Verification items for the finished model (mm, model axes). A direction names the side the tool comes from. Give positions to 0.01 mm unless a question says otherwise; leave off trailing zeros. Order: outer loops, then holes, each group sorted by start corner. A loop starts at its lowest first (then second) coordinate and runs counter-clockwise, first axis right, second up. Notation, with made-up numbers: (83.5, 1.5) - (114.5, 1.5) arc R31 cw to (114.5, 31.5) - close; hole circle Ø11 at (-39, -27). An arc over 180 degrees is marked (long way). Answer as a JSON object with one key per item and string values.
```python
from build123d import *

# Parameters (mm, degrees)
F0_R     = 28.25
F0_R_2   = 27.05
F1_DEPTH = 8
F0_R_3   = 32.25
F0_R_4   = 4.8
F0_R_5   = 4
F2_DEPTH = 0.7
F3_DEPTH = 30
F4_R     = 0.6


with BuildPart() as f1:
    # F0 (on Top) → F1 (new body)
    with BuildSketch(Plane.XY):
        Circle(F0_R)
        Circle(F0_R_2, mode=Mode.SUBTRACT)
    extrude(amount=F1_DEPTH)

    # F0 (on Top) → F2 (join)
    with BuildSketch(Plane.XY):
        Circle(F0_R_3)
        Circle(F0_R, mode=Mode.SUBTRACT)
        Circle(F0_R)
        Circle(F0_R_2, mode=Mode.SUBTRACT)
        Circle(F0_R_2)
        Circle(F0_R_4, mode=Mode.SUBTRACT)
        Circle(F0_R_4)
        Circle(F0_R_5, mode=Mode.SUBTRACT)
    extrude(amount=-F2_DEPTH)

    # F0 (on Top) → F3 (join)
    with BuildSketch(Plane.XY):
        Circle(F0_R_4)
        Circle(F0_R_5, mode=Mode.SUBTRACT)
    extrude(amount=F3_DEPTH)

    # F4
    f4_edges = [f1.edges().sort_by_distance(p)[0] for p in [
        (-28.25, 0, 0),
        (-27.05, 0, 0),
        (-4.8, 0, 0),
    ]]
    fillet(f4_edges, radius=F4_R)


solid = f1.part
```
(1) Section check C-C (z = 2). Record the cut outline in (x, y).
Computed values:
{"outline": "circle Ø56.5 at (0, 0); circle Ø9.6 at (0, 0); hole circle Ø54.1 at (0, 0); hole circle Ø8 at (0, 0)"}
(2) Material ranges on line 1 along Y through (x, z) = (0, 2.5); line 2 along Y through (x, z) = (0, 21); line 3 along Z through (x, y) = (12, -6), recorded low to high. Write a range as [from, to].
Computed values:
{"line 1": "y = [-28.25, -27.05], [-4.8, -4], [4, 4.8], [27.05, 28.25]", "line 2": "y = [-4.8, -4], [4, 4.8]", "line 3": "z = [-0.7, 0]"}
(3) Release check for a two-part mould opening along X. For faces 1 (the cylindrical face through (-0.867, -3.905, 14.435)), 2 (the flat face through (23, -15, 8)), 3 (the cylindrical face through (15.19, 23.82, 4.25)) record: pulls with the +X half, pulls with the -X half, needs draft (parallel to the pull), parting line crosses it, or undercut.
Computed values:
{"face 1": "undercut", "face 2": "needs draft", "face 3": "parting line crosses it"}
(4) Section check D-D (z = 24). Record the cut outline in (x, y).
Computed values:
{"outline": "circle Ø9.6 at (0, 0); hole circle Ø8 at (0, 0)"}
(5) Section check A-A (y = 0). Record the cut outline in (x, z).
Computed values:
{"outline": "(-32.25, -0.7) - (-4, -0.7) - (-4, 30) - (-4.8, 30) - (-4.8, 0.6) arc R0.6 cw to (-5.4, 0) - (-26.45, 0) arc R0.6 cw to (-27.05, 0.6) - (-27.05, 8) - (-28.25, 8) - (-28.25, 0.6) arc R0.6 cw to (-28.85, 0) - (-32.25, 0) - close; (4, -0.7) - (32.25, -0.7) - (32.25, 0) - (28.85, 0) arc R0.6 cw to (28.25, 0.6) - (28.25, 8) - (27.05, 8) - (27.05, 0.6) arc R0.6 cw to (26.45, 0) - (5.4, 0) arc R0.6 cw to (4.8, 0.6) - (4.8, 30) - (4, 30) - close"}
(6) Gauge pin test, flat ends, axial feed: pin 1 Ø6.5 at (x, y) = (0, 0) entering from +Z; pin 2 Ø10 at (x, y) = (23, -24.5) entering from -Z; pin 3 Ø12 at (y, z) = (9.5, 17) entering from +X; pin 4 Ø10 at (x, y) = (8, -25) entering from +Z. Record the tip position at first contact, or that the pin passes through.
Computed values:
{"pin 1": "passes through", "pin 2": "stops at z = -0.7", "pin 3": "stops at x = 3.28", "pin 4": "stops at z = 8"}
(7) Access from +Z, -Z, +X, -X, +Y, -Y to the whole of each face (thin tool, end or side, straight path). Record for faces 4 (the cylindrical face through (30.76, 9.69, -0.35)), 5 (the cylindrical face through (-21.466, -16.46, 4.248)).
Computed values:
{"face 4": "+Z, -Z", "face 5": "+Z"}
